Part model, mm, in its own coordinate system. Face numbers are marked on the shaded views. Give positions to 0.01 mm unless a question says otherwise; leave off trailing zeros. Order: outer loops, then holes, each group sorted by start corner. A loop starts at its lowest first (then second) coordinate and runs counter-clockwise, first axis right, second up. Notation, with made-up numbers: (32.5, 32.5) -> (86.5, 32.5) arc R14 cw to (86.5, 36.5) -> close; hole circle Ø6 at (40, 26.5). An arc over 180 degrees is marked (long way). Write item = value, one per line. Start each with the question number.
Item 1: Drill centre lines: line 1 along Z through (x, y) = (1.95, 6.9) (3 decimals); line 2 along Y through (x, z) = (1.25, 11.25); line 3 along Y through (x, z) = (0.65, 9.75). Where is each one in solid material? Low to high.
Item 2: Band-saw the part on B-B on x = 2.2. Count the separate pieces of the cut face and the enclosed holes in it, plus the area to 3 significant figures.
Item 3: Pull direction Z, two halves, no side cores. Call the marked faces 1, 2 and 3: +Z half, -Z half, draft (parallel to the pull), parting line (faces both ways), or undercut.
Item 4: Band-saw the part on A-A on y = -5.1. Write the cut outline in (x, z) (3 decimals), plus the area to 4 significant figures.
Autodesk Inventor part; units mm, degrees
ref_plane "YZ Plane" through (0, 0, 0) normal (1, 0, 0) x (0, 1, 0)
ref_plane "XZ Plane" through (0, 0, 0) normal (0, 1, 0) x (-1, 0, 0)
ref_plane "XY Plane" through (0, 0, 0) normal (0, 0, 1) x (1, 0, 0)
sketch "Sketch1" plane through (0, 0, 0) normal (1, 0, 0) x (0, 1, 0)
  line L0 (11.1, 12.625) -> (-11.1, 12.625)
  line L1 (-11.1, 12.625) -> (-11.1, -12.625)
  line L2 (-11.1, -12.625) -> (11.1, -12.625)
  line L3 (11.1, -12.625) -> (11.1, 12.625)
  line L4 (7.1853, 0) -> (-6.35, 0) construction
  line L5 (0, 7.4808) -> (0, -6.6937) construction
  circle A0 centre (-5.1, 10.375) radius 1
  circle A1 centre (-5.1, 2.625) radius 1
  circle A2 centre (-5.1, -10.375) radius 1
  circle A3 centre (-5.1, -2.625) radius 1
  circle A4 centre (6.9, 10.375) radius 1
  circle A5 centre (6.9, -10.375) radius 1
  circle A6 centre (6.9, 2.625) radius 1
  circle A7 centre (6.9, -2.625) radius 1
  point P0 (0, 0)
  dimension "d0" = 22.2
  dimension "d1" = 25.25
  dimension "d2" = 2
  dimension "d3" = 6
  dimension "d4" = 2.25
  dimension "d5" = 2
  dimension "d6" = 10
  dimension "d9" = 2
  dimension "d10" = 4.2
  dimension "d14" = 2
  dimension "d15" = 2
extrude "Extrusion1" add sketch "Sketch1" along normal blind 3 contours L3 L2 L1 L0 | A6 | A7
extrude "Extrusion2" cut sketch "Sketch1" along normal blind 3 contours A6 | A7
properties part number "Konektor Lifter_3DPrint"
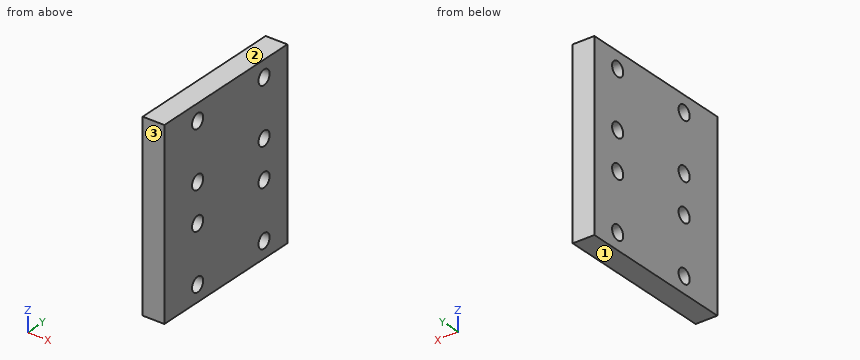
Values found:
q1.line_1 = -12.625 to -11.375, -9.375 to -3.625, -1.625 to 1.625, 3.625 to 9.375, 11.375 to 12.625
q1.line_2 = -11.1 to -5.58, -4.62 to 6.42, 7.38 to 11.1
q1.line_3 = -11.1 to -5.88, -4.32 to 6.12, 7.68 to 11.1
q2.separate_pieces = 1
q2.enclosed_holes = 8
q2.area = 535 mm^2
q3.face_1 = -Z half
q3.face_2 = +Z half
q3.face_3 = draft
q4.outline = (0, -12.625) -> (3, -12.625) -> (3, -11.375) -> (0, -11.375) -> close; (0, -9.375) -> (3, -9.375) -> (3, -3.625) -> (0, -3.625) -> close; (0, -1.625) -> (3, -1.625) -> (3, 1.625) -> (0, 1.625) -> close; (0, 3.625) -> (3, 3.625) -> (3, 9.375) -> (0, 9.375) -> close; (0, 11.375) -> (3, 11.375) -> (3, 12.625) -> (0, 12.625) -> close
q4.area = 51.75 mm^2
